The listing builds one solid part. Answer for the finished solid, in the listing's coordinates (mm). Face numbers are marked on the shaded views. A direction names the side the tool comes from. Round coordinates to 2 decimals unless told otherwise and drop trailing zeros. Write each loop counter-clockwise with the first axis right and the second up, starting at its lowest first coordinate (ties: lowest second). Pieces come first, ordered by that corner, then holes. Notation, with made-up numbers: M 53,33 L 106,33 A29 cw 106,56 Z; hole C 74.25,48 d10. An arc over 180 degrees is marked long. One line per item, written item: value. Start each with the question number.
(1) Consider probe 1 along X at (y, z) = (3.75, 0); probe 2 along Y at (x, z) = (-27, -3.5); probe 3 along Z at (x, y) = (-11, 4.25). Determine where each line is inside the solid, lowest interval first.
(2) Section C-C (x = 14.5) is taken. Determine the outline of the cut face in (y, z).
(3) Section A-A (z = 0) is taken. Determine the outline of the cut face in (x, y).
(4) For a pull along Y with two mould halves and no side action, classify the marked faces 1, 2 and 3 as released by +Y, released by -Y, zero draft, split by the parting line, or undercut.
(5) For the marked faces 4, 5 and 6, determine the directions among +Z, -Z, +X, -X, +Y, -Y from which every point of the face is accessible in a straight line to the end or side of a thin tool.
(6) Section D-D (z = 14) is taken. Determine the outline of the cut face in (x, y), plus the area to 3 significant figures.
(7) Given P1, Ø2, axis at y = 3.5, z = 1, coming from the +X side; P2, Ø1.5, axis at x = 14, y = 3, coming from the -Z side; P3, Ø5, axis at y = 3, z = -18, coming from the +X side; P4, Ø13.5, axis at x = 0, z = 0, coming from the +Y side, each flat-ended and moving along its own axis, determine where each tip first touches the part or whether it passes through.
(8) Section B-B (y = 5.25) is taken. Determine the outline of the cut face in (x, z) (3 decimals), plus the area to 3 significant figures.
```python
from build123d import *

# Parameters (mm, degrees)
SKETCH3_R                     = 0.25
BOSS_EXTRUDE1_DEPTH           = 7
BOSS_EXTRUDE1_DRAFT           = 0.5
BOSS_EXTRUDE1_PROFILE_2_DEPTH = 7
BOSS_EXTRUDE1_PROFILE_2_DRAFT = 0.5
BOSS_EXTRUDE1_PROFILE_3_DEPTH = 7
BOSS_EXTRUDE1_PROFILE_3_DRAFT = 0.5
BOSS_EXTRUDE1_PROFILE_4_DEPTH = 7
BOSS_EXTRUDE1_PROFILE_4_DRAFT = 0.5
BOSS_EXTRUDE1_PROFILE_5_DEPTH = 7
BOSS_EXTRUDE1_PROFILE_5_DRAFT = 0.5
BOSS_EXTRUDE1_PROFILE_6_DEPTH = 7
BOSS_EXTRUDE1_PROFILE_6_DRAFT = 0.5


with BuildPart() as part:
    # Sketch2 → Revolve1 (revolve)
    with BuildSketch(Plane.XY, mode=Mode.PRIVATE) as revolve1_sk:
        Polygon((-8.55, 0), (-30, 0), (-30, 2), (-16.15, 2), (-16.15, 3), (-12.65, 3), (-12.65, 10), (-8.55, 10), align=None)
    revolve(revolve1_sk.sketch.rotate(Axis((0, 0, 0), (0, 1, 0)), 270), axis=Axis((0, 0, 0), (0, 1, 0)))


with BuildPart() as boss_extrude1_tool:
    # Sketch3 → Boss-Extrude1 (with draft: the straight prism first)
    with BuildSketch(Plane(origin=(0, 3, 0), x_dir=(1, 0, 0), z_dir=(0, 1, 0))):
        with Locations((0, 12.55)):
            Circle(SKETCH3_R)
    extrude(amount=BOSS_EXTRUDE1_DEPTH)
    # Boss-Extrude1: the draft: its side faces are tilted about the plane it starts from
    boss_extrude1_sides = [boss_extrude1_tool.faces().sort_by_distance(p)[0] for p in [
        (-0.25, 6.5, -12.55),
    ]]
    draft(boss_extrude1_sides, Plane(origin=(0, 3, 0), x_dir=(1, 0, 0), z_dir=(0, 1, 0)), BOSS_EXTRUDE1_DRAFT)


with BuildPart() as part_1:
    add(part.part)

    # Boss-Extrude1: add boss_extrude1_tool
    add(boss_extrude1_tool.part)


with BuildPart() as boss_extrude1_profile_2_tool:
    # Sketch3 → Boss-Extrude1 profile 2 (with draft: the straight prism first)
    with BuildSketch(Plane(origin=(0, 3, 0), x_dir=(1, 0, 0), z_dir=(0, 1, 0))):
        with Locations((10.868618817, 6.275)):
            Circle(SKETCH3_R)
    extrude(amount=BOSS_EXTRUDE1_PROFILE_2_DEPTH)
    # Boss-Extrude1 profile 2: the draft: its side faces are tilted about the plane it starts from
    boss_extrude1_profile_2_sides = [boss_extrude1_profile_2_tool.faces().sort_by_distance(p)[0] for p in [
        (10.618618817, 6.5, -6.275),
    ]]
    draft(boss_extrude1_profile_2_sides, Plane(origin=(0, 3, 0), x_dir=(1, 0, 0), z_dir=(0, 1, 0)), BOSS_EXTRUDE1_PROFILE_2_DRAFT)


with BuildPart() as part_2:
    add(part_1.part)

    # Boss-Extrude1 profile 2: add boss_extrude1_profile_2_tool
    add(boss_extrude1_profile_2_tool.part)


with BuildPart() as boss_extrude1_profile_3_tool:
    # Sketch3 → Boss-Extrude1 profile 3 (with draft: the straight prism first)
    with BuildSketch(Plane(origin=(0, 3, 0), x_dir=(1, 0, 0), z_dir=(0, 1, 0))):
        with Locations((10.868618817, -6.275)):
            Circle(SKETCH3_R)
    extrude(amount=BOSS_EXTRUDE1_PROFILE_3_DEPTH)
    # Boss-Extrude1 profile 3: the draft: its side faces are tilted about the plane it starts from
    boss_extrude1_profile_3_sides = [boss_extrude1_profile_3_tool.faces().sort_by_distance(p)[0] for p in [
        (10.618618817, 6.5, 6.275),
    ]]
    draft(boss_extrude1_profile_3_sides, Plane(origin=(0, 3, 0), x_dir=(1, 0, 0), z_dir=(0, 1, 0)), BOSS_EXTRUDE1_PROFILE_3_DRAFT)


with BuildPart() as part_3:
    add(part_2.part)

    # Boss-Extrude1 profile 3: add boss_extrude1_profile_3_tool
    add(boss_extrude1_profile_3_tool.part)


with BuildPart() as boss_extrude1_profile_4_tool:
    # Sketch3 → Boss-Extrude1 profile 4 (with draft: the straight prism first)
    with BuildSketch(Plane(origin=(0, 3, 0), x_dir=(1, 0, 0), z_dir=(0, 1, 0))):
        with Locations((0, -12.55)):
            Circle(SKETCH3_R)
    extrude(amount=BOSS_EXTRUDE1_PROFILE_4_DEPTH)
    # Boss-Extrude1 profile 4: the draft: its side faces are tilted about the plane it starts from
    boss_extrude1_profile_4_sides = [boss_extrude1_profile_4_tool.faces().sort_by_distance(p)[0] for p in [
        (-0.25, 6.5, 12.55),
    ]]
    draft(boss_extrude1_profile_4_sides, Plane(origin=(0, 3, 0), x_dir=(1, 0, 0), z_dir=(0, 1, 0)), BOSS_EXTRUDE1_PROFILE_4_DRAFT)


with BuildPart() as part_4:
    add(part_3.part)

    # Boss-Extrude1 profile 4: add boss_extrude1_profile_4_tool
    add(boss_extrude1_profile_4_tool.part)


with BuildPart() as boss_extrude1_profile_5_tool:
    # Sketch3 → Boss-Extrude1 profile 5 (with draft: the straight prism first)
    with BuildSketch(Plane(origin=(0, 3, 0), x_dir=(1, 0, 0), z_dir=(0, 1, 0))):
        with Locations((-10.868618817, -6.275)):
            Circle(SKETCH3_R)
    extrude(amount=BOSS_EXTRUDE1_PROFILE_5_DEPTH)
    # Boss-Extrude1 profile 5: the draft: its side faces are tilted about the plane it starts from
    boss_extrude1_profile_5_sides = [boss_extrude1_profile_5_tool.faces().sort_by_distance(p)[0] for p in [
        (-11.118618817, 6.5, 6.275),
    ]]
    draft(boss_extrude1_profile_5_sides, Plane(origin=(0, 3, 0), x_dir=(1, 0, 0), z_dir=(0, 1, 0)), BOSS_EXTRUDE1_PROFILE_5_DRAFT)


with BuildPart() as part_5:
    add(part_4.part)

    # Boss-Extrude1 profile 5: add boss_extrude1_profile_5_tool
    add(boss_extrude1_profile_5_tool.part)


with BuildPart() as boss_extrude1_profile_6_tool:
    # Sketch3 → Boss-Extrude1 profile 6 (with draft: the straight prism first)
    with BuildSketch(Plane(origin=(0, 3, 0), x_dir=(1, 0, 0), z_dir=(0, 1, 0))):
        with Locations((-10.868618817, 6.275)):
            Circle(SKETCH3_R)
    extrude(amount=BOSS_EXTRUDE1_PROFILE_6_DEPTH)
    # Boss-Extrude1 profile 6: the draft: its side faces are tilted about the plane it starts from
    boss_extrude1_profile_6_sides = [boss_extrude1_profile_6_tool.faces().sort_by_distance(p)[0] for p in [
        (-11.118618817, 6.5, -6.275),
    ]]
    draft(boss_extrude1_profile_6_sides, Plane(origin=(0, 3, 0), x_dir=(1, 0, 0), z_dir=(0, 1, 0)), BOSS_EXTRUDE1_PROFILE_6_DRAFT)


with BuildPart() as part_6:
    add(part_5.part)

    # Boss-Extrude1 profile 6: add boss_extrude1_profile_6_tool
    add(boss_extrude1_profile_6_tool.part)


solid = part_6.part
```
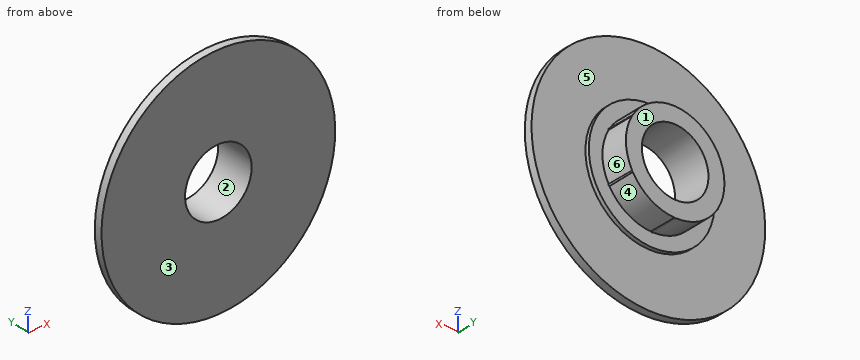
Recorded:
1. probe 1: x = -12.65 to -8.55, 8.55 to 12.65
1. probe 2: y = 0 to 2
1. probe 3: z = -6.47 to 6.47
2. outline: M 0,-26.26 L 2,-26.26 L 2,-7.11 L 3,-7.11 L 3,7.11 L 2,7.11 L 2,26.26 L 0,26.26 Z
3. outline: M -30,0 L -8.55,0 L -8.55,10 L -12.65,10 L -12.65,3 L -16.15,3 L -16.15,2 L -30,2 Z; M 8.55,0 L 30,0 L 30,2 L 16.15,2 L 16.15,3 L 12.65,3 L 12.65,10 L 8.55,10 Z
4. face 1: released by +Y
4. face 2: zero draft
4. face 3: released by -Y
5. face 4: -Z, +X, +Y
5. face 5: +Y
5. face 6: +X, +Y
6. outline: M -26.53,0 L 26.53,0 L 26.53,2 L 8.05,2 L 8.05,3 L -8.05,3 L -8.05,2 L -26.53,2 Z
6. area: 122 mm2
7. P1: stops at x = 16.15
7. P2: stops at z = -9.23
7. P3: stops at x = 25.56
7. P4: passes through
8. outline: M -11.058,-6.144 A0.23 ccw -10.85,-6.505 A12.65 ccw -0.208,-12.648 A0.23 ccw 0.208,-12.648 A12.65 ccw 10.85,-6.505 A0.23 ccw 11.058,-6.144 A12.65 ccw 11.058,6.144 A0.23 ccw 10.85,6.505 A12.65 ccw 0.208,12.648 A0.23 ccw -0.208,12.648 A12.65 ccw -10.85,6.505 A0.23 ccw -11.058,6.144 A12.65 ccw Z; hole C 0,0 d17.1
8. area: 273 mm2
